Geometry check sheet. Reference: the model listing, model coordinates, mm. Face numbers are marked on the shaded views. A direction names the side the tool comes from. Coordinates: 2 decimals unless noted, no trailing zeros. Loops run counter-clockwise (first coordinate to the right, second up) from the corner with the lowest first, then second, coordinate; pieces in that order, holes last. Notation, with made-up numbers: (80.5, 6.5) - (123.5, 6.5) arc R28 cw to (123.5, 44.5) - close; hole circle Ø2 at (48, 72.5). An arc over 180 degrees is marked (long way). Write each question's results on one line, items separated by ' | '. Start each with the question number.
(1) Mould release check, pull along X, two halves, no side actions. Record for the marked faces 1, 2 and 3: pulls with the +X half, pulls with the -X half, needs draft (parallel to the pull), parting line crosses it, or undercut.
(2) Sectioned sample at C-C (z = -25). Enter the section's corners in (x, y), plus the area to 3 significant figures.
(3) Sectioned sample at A-A (x = 37.5). Enter the section's corners in (y, z).
(4) Sectioned sample at D-D (y = 14). State how many separate pieces and enclosed holes the cut face has, plus the area to 3 significant figures.
(5) Sectioned sample at B-B (y = 2.25). Enter the section's corners in (x, z), plus the area to 3 significant figures.
(6) Access from +Z, -Z, +X, -X, +Y, -Y to the whole of each face (thin tool, end or side, straight path). Record for the marked faces 4, 5 and 6.
(7) Material ranges on probe 1 along Z at (x, y) = (37.5, 18.4); probe 2 along X at (y, z) = (18.4, -25); probe 3 along Z at (x, y) = (38, 5), recorded low to high.
(8) Go/stop test with flat-tipped pins: pin 1 Ø8 at (y, z) = (10, -10.5) entering from +X; pin 2 Ø1.5 at (y, z) = (8, -35.5) entering from -X; pin 3 Ø4 at (x, y) = (61, 3.5) entering from -Z. Record where each tip stops, or that it passes through.
from build123d import *

# Parameters (mm, degrees)
SKETCH1_W           = 75
SKETCH1_H           = 50
BOSS_EXTRUDE1_DEPTH = 20
SKETCH2_R           = 21
SKETCH2_R_2         = 16
CUT_EXTRUDE1_DEPTH  = 5
SKETCH3_W           = 14
SKETCH3_H           = 14
CUT_EXTRUDE2_DEPTH  = 21
CUT_EXTRUDE3_DEPTH  = 21
CUT_EXTRUDE6_DEPTH  = 10


with BuildPart() as part:
    # Sketch1 → Boss-Extrude1 (new body)
    with BuildSketch(Plane(origin=(0, 0, 0), x_dir=(1, 0, 0), z_dir=(0, 1, 0))):
        with Locations((37.5, 25)):
            Rectangle(SKETCH1_W, SKETCH1_H)
    extrude(amount=BOSS_EXTRUDE1_DEPTH)

    # Sketch2 → Cut-Extrude1 (cut)
    with BuildSketch(Plane(origin=(0, 20, 0), x_dir=(1, 0, 0), z_dir=(0, 1, 0))):
        with Locations((37.5, 25)):
            Circle(SKETCH2_R)
        with Locations((37.5, 25)):
            Circle(SKETCH2_R_2, mode=Mode.SUBTRACT)
    extrude(amount=-CUT_EXTRUDE1_DEPTH, mode=Mode.SUBTRACT)

    # Sketch3 → Cut-Extrude2 (cut, through all)
    with BuildSketch(Plane(origin=(0, 20, 0), x_dir=(1, 0, 0), z_dir=(0, 1, 0))):
        with Locations((37.5, 25)):
            Rectangle(SKETCH3_W, SKETCH3_H)
    extrude(amount=-CUT_EXTRUDE2_DEPTH, mode=Mode.SUBTRACT)

    # Sketch4 → Cut-Extrude3 (cut, through all)
    with BuildSketch(Plane.XZ):
        with BuildLine():
            Line((0, -29), (0, -50))
            Line((0, -50), (21, -50))
            ThreePointArc((21, -50), (14.849242405, -35.150757595), (0, -29))
        make_face()
        with BuildLine():
            Line((75, -29), (75, -50))
            Line((75, -50), (54, -50))
            ThreePointArc((54, -50), (60.150757595, -35.150757595), (75, -29))
        make_face()
        with BuildLine():
            Line((75, -21), (75, 0))
            Line((75, 0), (54, 0))
            ThreePointArc((54, 0), (60.150757595, -14.849242405), (75, -21))
        make_face()
        with BuildLine():
            Line((0, 0), (21, 0))
            ThreePointArc((21, 0), (14.849242405, -14.849242405), (0, -21))
            Line((0, -21), (0, 0))
        make_face()
    extrude(amount=-CUT_EXTRUDE3_DEPTH, mode=Mode.SUBTRACT)

    # Sketch6 → Cut-Extrude6 (cut)
    with BuildSketch(Plane(origin=(0, 20, 0), x_dir=(1, 0, 0), z_dir=(0, 1, 0))):
        with BuildLine():
            Line((30.6443454, 48), (22.912878475, 48))
            ThreePointArc((22.912878475, 48), (22.583722585, 45.643915266), (22.012955919, 43.334433878))
            ThreePointArc((22.012955919, 43.334433878), (26.087685471, 46.113007296), (30.6443454, 48))
        make_face()
        with BuildLine():
            Line((44.3556546, 2), (52.087121525, 2))
            ThreePointArc((52.087121525, 2), (52.416277415, 4.356084734), (52.987044081, 6.665566122))
            ThreePointArc((52.987044081, 6.665566122), (48.912314529, 3.886992704), (44.3556546, 2))
        make_face()
        with BuildLine():
            Line((2, 27.087121525), (2, 22.912878475))
            ThreePointArc((2, 22.912878475), (8.700524902, 21.29086345), (14.619351774, 17.755972339))
            ThreePointArc((14.619351774, 17.755972339), (13.5, 25), (14.619351774, 32.244027661))
            ThreePointArc((14.619351774, 32.244027661), (8.700524902, 28.70913655), (2, 27.087121525))
        make_face()
        with BuildLine():
            Line((22.912878475, 2), (30.6443454, 2))
            ThreePointArc((30.6443454, 2), (26.087685471, 3.886992704), (22.012955919, 6.665566122))
            ThreePointArc((22.012955919, 6.665566122), (22.583722585, 4.356084734), (22.912878475, 2))
        make_face()
        with BuildLine():
            Line((73, 22.912878475), (73, 27.087121525))
            ThreePointArc((73, 27.087121525), (66.299475098, 28.70913655), (60.380648226, 32.244027661))
            ThreePointArc((60.380648226, 32.244027661), (61.5, 25), (60.380648226, 17.755972339))
            ThreePointArc((60.380648226, 17.755972339), (66.299475098, 21.29086345), (73, 22.912878475))
        make_face()
        with BuildLine():
            Line((52.087121525, 48), (44.3556546, 48))
            ThreePointArc((44.3556546, 48), (48.912314529, 46.113007296), (52.987044081, 43.334433878))
            ThreePointArc((52.987044081, 43.334433878), (52.416277415, 45.643915266), (52.087121525, 48))
        make_face()
    extrude(amount=-CUT_EXTRUDE6_DEPTH, mode=Mode.SUBTRACT)


solid = part.part
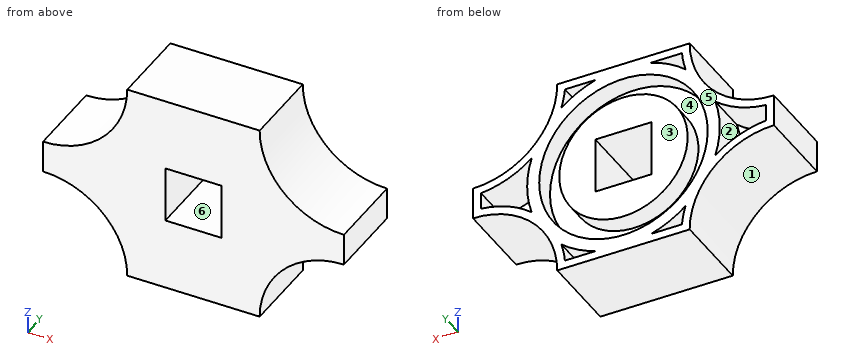
Outcome:
1) face 1: pulls with the -X half | face 2: undercut | face 3: needs draft
2) outline: (0, 0) - (30.5, 0) - (30.5, 20) - (21.5, 20) - (21.5, 15) - (16.5, 15) - (16.5, 20) - (13.5, 20) - (13.5, 10) - (2, 10) - (2, 20) - (0, 20) - close; (44.5, 0) - (75, 0) - (75, 20) - (73, 20) - (73, 10) - (61.5, 10) - (61.5, 20) - (58.5, 20) - (58.5, 15) - (53.5, 15) - (53.5, 20) - (44.5, 20) - close | area: 940 mm2
3) outline: (0, -50) - (20, -50) - (20, -46) - (15, -46) - (15, -41) - (20, -41) - (20, -32) - (0, -32) - close; (0, -18) - (20, -18) - (20, -9) - (15, -9) - (15, -4) - (20, -4) - (20, 0) - (0, 0) - close
4) separate pieces: 1 | enclosed holes: 7 | area: 1,940 mm2
5) outline: (0, -29) arc R21 cw to (21, -50) - (54, -50) arc R21 cw to (75, -29) - (75, -21) arc R21 cw to (54, 0) - (21, 0) arc R21 cw to (0, -21) - close; hole (30.5, -32) - (44.5, -32) - (44.5, -18) - (30.5, -18) - close | area: 2,170 mm2
6) face 4: +Y | face 5: +Z, -Z, +X, -X, +Y | face 6: +Y, -Y
7) probe 1: z = -50 to -46, -41 to -32, -18 to -9, -4 to 0 | probe 2: x = 0 to 2, 13.5 to 16.5, 21.5 to 30.5, 44.5 to 53.5, 58.5 to 61.5, 73 to 75 | probe 3: z = -50 to -32, -18 to 0
8) pin 1: stops at x = 59.81 | pin 2: stops at x = 14.44 | pin 3: stops at z = -36.4
